The listing builds one solid part. Answer for the finished solid, in the listing's coordinates (mm). A direction names the side the tool comes from. Round coordinates to 2 decimals unless told otherwise and drop trailing zeros. Order: outer loops, then holes, each group sorted by start corner. A loop starts at its lowest first (then second) coordinate and runs counter-clockwise, first axis right, second up. Notation, with made-up numbers: M 56,82 L 67,82 A22 cw 67,99 Z; hole C 22,-8.5 d6. An arc over 180 degrees is marked long. Write item = value, one per line. Start each with the question number.
(1) For a pull along Y with two mould halves and no side action, classify faces 4 (the face through (0, 106, 2)), 5 (the face through (0, -5, 0)), 6 (the face through (-3, 0, 3)), 7 (the face through (3.746, 49.51, 0.165)) as released by +Y, released by -Y, zero draft, split by the parting line, or undercut.
(2) A cutting plane is placed at A-A, the plane z = 0. Determine the outline of the cut face in (x, y), and give its area (3 significant figures).
(3) Each of these flat-tipped pins is pushed along its axis until it touches: pin 1 (14.5 mm diameter, centred on x = 1, z = -3.5, fed in from -Y); pin 2 (1.5 mm diameter, centred on x = 0.5, y = 63, fed in from +Z); pin 3 (3 mm diameter, centred on x = -1.5, z = -3.5, fed in from -Y); pin 4 (5 mm diameter, centred on y = 36, z = -1.5, fed in from +X). Where does it stop, or does it pass through?
(4) Straight lines are drawn through the part: probe 1 along Z at (x, y) = (0, -18); probe 2 along X at (y, z) = (69.5, -0.25); probe 3 along Y at (x, z) = (4.5, 3). For each, find the intervals that lie inside material, in ascending order. Write a range as from..to.
(5) Which of the six approach directions +Z, -Z, +X, -X, +Y, -Y give full straight-line access (tool end or side, diameter ignored) to faces 1 (the face through (-1.172, -13.874, 8.923)), 2 (the face through (0.867, 91.902, -3.905)), 3 (the face through (0, 114, 0))?
(6) A cutting plane is placed at D-D, the plane y = 28. Determine the outline of the cut face in (x, z), and give its area (3 significant figures).
(7) A cutting plane is placed at B-B, the plane x = 0. Determine the outline of the cut face in (y, z), and give its area (3 significant figures).
(8) A cutting plane is placed at C-C, the plane y = 2. Determine the outline of the cut face in (x, z), and give its area (3 significant figures).
from build123d import *

# Parameters (mm, degrees)
F0_R      = 12.5
F1_DEPTH  = 5
F2_R      = 12.5
F2_R_2    = 9
F3_DEPTH  = 18
F4_R      = 4
F5_DEPTH  = 15
F6_R      = 3.75
F7_DEPTH  = 70
F8_R      = 4
F9_DEPTH  = 14
F11_DEPTH = 15


with BuildPart() as f1:
    # F0 (on Front) → F1 (new body)
    with BuildSketch(Plane.XZ):
        Circle(F0_R)
    extrude(amount=F1_DEPTH)

    # F2 (on face) → F3 (join)
    with BuildSketch(Plane.XZ.offset(5)):
        Circle(F2_R)
        Circle(F2_R_2, mode=Mode.SUBTRACT)
    extrude(amount=F3_DEPTH)

    # F4 (on face) → F5 (join)
    with BuildSketch(Plane(origin=(0, 0, 0), x_dir=(-1, 0, 0), z_dir=(0, 1, 0))):
        Circle(F4_R)
    extrude(amount=F5_DEPTH)

    # F6 (on face) → F7 (join)
    with BuildSketch(Plane(origin=(0, 15, 0), x_dir=(-1, 0, 0), z_dir=(0, 1, 0))):
        Circle(F6_R)
    extrude(amount=F7_DEPTH)

    # F8 (on face) → F9 (join)
    with BuildSketch(Plane(origin=(0, 85, 0), x_dir=(-1, 0, 0), z_dir=(0, 1, 0))):
        Circle(F8_R)
    extrude(amount=F9_DEPTH)

    # F10 (on face) → F11 (join)
    with BuildSketch(Plane(origin=(0, 99, 0), x_dir=(-1, 0, 0), z_dir=(0, 1, 0))):
        with BuildLine():
            Line((2.236068, 2), (-2.236068, 2))
            ThreePointArc((-2.236068, 2), (0, -3), (2.236068, 2))
        make_face()
    extrude(amount=F11_DEPTH)


solid = f1.part
Reported:
q1.face_4 = zero draft
q1.face_5 = released by -Y
q1.face_6 = released by +Y
q1.face_7 = undercut
q2.outline = M -12.5,-23 L -9,-23 L -9,-5 L 9,-5 L 9,-23 L 12.5,-23 L 12.5,0 L 4,0 L 4,15 L 3.75,15 L 3.75,85 L 4,85 L 4,99 L 3,99 L 3,114 L -3,114 L -3,99 L -4,99 L -4,85 L -3.75,85 L -3.75,15 L -4,15 L -4,0 L -12.5,0 Z
q2.area = 1,100 mm²
q3.pin_1 = -23
q3.pin_2 = 3.75
q3.pin_3 = -5
q3.pin_4 = 3.75
q4.probe_1 = -12.5..-9, 9..12.5
q4.probe_2 = -3.74..3.74
q4.probe_3 = -5..0
q5.face_1 = -Y
q5.face_2 = +Y
q5.face_3 = +Z, -Z, +X, -X, +Y
q6.outline = C 0,0 d7.5
q6.area = 44.2 mm²
q7.outline = M -23,-12.5 L 0,-12.5 L 0,-4 L 15,-4 L 15,-3.75 L 85,-3.75 L 85,-4 L 99,-4 L 99,-3 L 114,-3 L 114,2 L 99,2 L 99,4 L 85,4 L 85,3.75 L 15,3.75 L 15,4 L 0,4 L 0,12.5 L -23,12.5 L -23,9 L -5,9 L -5,-9 L -23,-9 Z
q7.area = 1,080 mm²
q8.outline = C 0,0 d8
q8.area = 50.3 mm²
